Work out the finished part from the listing and answer in its coordinate system (mm). A direction names the side the tool comes from. Round coordinates to 2 decimals unless told otherwise and drop trailing zeros. Loops run counter-clockwise (first coordinate to the right, second up) from the corner with the lowest first, then second, coordinate; pieces in that order, holes last. Notation, with made-up numbers: (23, -3.5) - (45, -3.5) arc R14 cw to (45, 22.5) - close; hole circle Ø10 at (54.5, -16.5). An arc over 180 degrees is marked (long way). Answer as CSV lines item,"result". Start each with the question number.
```python
from build123d import *

# Parameters (mm, degrees)
SKETCH1_R               = 63.5
BOSS_EXTRUDE1_DEPTH     = 25.4
SKETCH2_W               = 190.5
SKETCH2_H               = 190.5
BOSS_EXTRUDE2_DEPTH     = 990.6
BOSS_EXTRUDE3_START     = 25.4
SKETCH3_R               = 63.5
BOSS_EXTRUDE3_DEPTH     = 25.4
SKETCH4_W               = 38.1
SKETCH4_H               = 200.66
BOSS_EXTRUDE4_DEPTH     = 10.16
SKETCH5_R               = 9.525
BOSS_EXTRUDE5_DEPTH     = 4.445
CIRPATTERN3_COUNT       = 4
MIRROR1_COPY_1_SKETCH_W = 38.1
MIRROR1_COPY_1_SKETCH_H = 200.66
MIRROR1_COPY_1_DEPTH    = 10.16
MIRROR1_COPY_2_SKETCH_W = 38.1
MIRROR1_COPY_2_SKETCH_H = 200.66
MIRROR1_COPY_2_DEPTH    = 10.16
MIRROR1_COPY_3_SKETCH_W = 38.1
MIRROR1_COPY_3_SKETCH_H = 200.66
MIRROR1_COPY_3_DEPTH    = 10.16
MIRROR1_COPY_4_SKETCH_R = 9.525
MIRROR1_COPY_4_DEPTH    = 4.445
MIRROR1_COPY_5_SKETCH_R = 9.525
MIRROR1_COPY_5_DEPTH    = 4.445
MIRROR1_COPY_6_SKETCH_R = 9.525
MIRROR1_COPY_6_DEPTH    = 4.445


with BuildPart() as part:
    # Sketch1 → Boss-Extrude1 (new body)
    with BuildSketch(Plane.XY):
        Circle(SKETCH1_R)
    extrude(amount=BOSS_EXTRUDE1_DEPTH)

    # Sketch2 → Boss-Extrude2 (add)
    with BuildSketch(Plane(origin=(0, 0, 0), x_dir=(-1, 0, 0), z_dir=(0, 0, -1))):
        Rectangle(SKETCH2_W, SKETCH2_H)
    extrude(amount=BOSS_EXTRUDE2_DEPTH)

    # Sketch3 → Boss-Extrude3 (add)
    with BuildSketch(Plane(origin=(0, 0, -990.6), x_dir=(-1, 0, 0), z_dir=(0, 0, -1)).offset(BOSS_EXTRUDE3_START)):
        with Locations(Location((0, 0, 0), (0, 0, 180))):
            Circle(SKETCH3_R)
    extrude(amount=-BOSS_EXTRUDE3_DEPTH)

    # Sketch4 → Boss-Extrude4 (add)
    with BuildSketch(Plane(origin=(95.25, 0, 0), x_dir=(0, 0, -1), z_dir=(1, 0, 0))):
        with Locations((31.75, 5.08)):
            Rectangle(SKETCH4_W, SKETCH4_H)
    boss_extrude4 = extrude(amount=BOSS_EXTRUDE4_DEPTH)

    # Sketch5 → Boss-Extrude5 (add)
    with BuildSketch(Plane(origin=(105.41, 0, 0), x_dir=(0, 0, -1), z_dir=(1, 0, 0))):
        with Locations(Location((31.75, 82.55, 0), (0, 0, 180))):
            Circle(SKETCH5_R)
        with Locations(Location((31.75, 41.91, 0), (0, 0, 180))):
            Circle(SKETCH5_R)
        with Locations(Location((31.75, 1.27, 0), (0, 0, 180))):
            Circle(SKETCH5_R)
        with Locations(Location((31.75, -39.37, 0), (0, 0, 180))):
            Circle(SKETCH5_R)
        with Locations(Location((31.75, -80.01, 0), (0, 0, 180))):
            Circle(SKETCH5_R)
    boss_extrude5 = extrude(amount=BOSS_EXTRUDE5_DEPTH)

    # CirPattern3: Boss-Extrude4, Boss-Extrude5 ×4 about axis
    cirpattern3_axis = Axis((0, 0, 0), (0, 0, 1))
    add([boss_extrude4.rotate(cirpattern3_axis, i * 360 / CIRPATTERN3_COUNT) for i in range(1, CIRPATTERN3_COUNT)])
    add([boss_extrude5.rotate(cirpattern3_axis, i * 360 / CIRPATTERN3_COUNT) for i in range(1, CIRPATTERN3_COUNT)])

    # Mirror1: Boss-Extrude4, Boss-Extrude5 across plane
    add(boss_extrude4.mirror(Plane.XY.offset(-495.3)))
    add(boss_extrude5.mirror(Plane.XY.offset(-495.3)))

    # Mirror1 copy 1 sketch → Mirror1 copy 1 (add)
    with BuildSketch(Plane(origin=(0, 95.25, -990.6), x_dir=(0, 0, 1), z_dir=(0, 1, 0))):
        with Locations((31.75, -5.08)):
            Rectangle(MIRROR1_COPY_1_SKETCH_W, MIRROR1_COPY_1_SKETCH_H)
    extrude(amount=MIRROR1_COPY_1_DEPTH)

    # Mirror1 copy 2 sketch → Mirror1 copy 2 (add)
    with BuildSketch(Plane(origin=(-95.25, 0, -990.6), x_dir=(0, 0, 1), z_dir=(-1, 0, 0))):
        with Locations((31.75, -5.08)):
            Rectangle(MIRROR1_COPY_2_SKETCH_W, MIRROR1_COPY_2_SKETCH_H)
    extrude(amount=MIRROR1_COPY_2_DEPTH)

    # Mirror1 copy 3 sketch → Mirror1 copy 3 (add)
    with BuildSketch(Plane(origin=(0, -95.25, -990.6), x_dir=(0, 0, 1), z_dir=(0, -1, 0))):
        with Locations((31.75, -5.08)):
            Rectangle(MIRROR1_COPY_3_SKETCH_W, MIRROR1_COPY_3_SKETCH_H)
    extrude(amount=MIRROR1_COPY_3_DEPTH)

    # Mirror1 copy 4 sketch → Mirror1 copy 4 (add)
    with BuildSketch(Plane(origin=(0, 105.41, -990.6), x_dir=(0, 0, 1), z_dir=(0, 1, 0))):
        with Locations((31.75, -82.55)):
            Circle(MIRROR1_COPY_4_SKETCH_R)
        with Locations((31.75, -41.91)):
            Circle(MIRROR1_COPY_4_SKETCH_R)
        with Locations((31.75, -1.27)):
            Circle(MIRROR1_COPY_4_SKETCH_R)
        with Locations((31.75, 39.37)):
            Circle(MIRROR1_COPY_4_SKETCH_R)
        with Locations((31.75, 80.01)):
            Circle(MIRROR1_COPY_4_SKETCH_R)
    extrude(amount=MIRROR1_COPY_4_DEPTH)

    # Mirror1 copy 5 sketch → Mirror1 copy 5 (add)
    with BuildSketch(Plane(origin=(-105.41, 0, -990.6), x_dir=(0, 0, 1), z_dir=(-1, 0, 0))):
        with Locations((31.75, -82.55)):
            Circle(MIRROR1_COPY_5_SKETCH_R)
        with Locations((31.75, -41.91)):
            Circle(MIRROR1_COPY_5_SKETCH_R)
        with Locations((31.75, -1.27)):
            Circle(MIRROR1_COPY_5_SKETCH_R)
        with Locations((31.75, 39.37)):
            Circle(MIRROR1_COPY_5_SKETCH_R)
        with Locations((31.75, 80.01)):
            Circle(MIRROR1_COPY_5_SKETCH_R)
    extrude(amount=MIRROR1_COPY_5_DEPTH)

    # Mirror1 copy 6 sketch → Mirror1 copy 6 (add)
    with BuildSketch(Plane(origin=(0, -105.41, -990.6), x_dir=(0, 0, 1), z_dir=(0, -1, 0))):
        with Locations((31.75, -82.55)):
            Circle(MIRROR1_COPY_6_SKETCH_R)
        with Locations((31.75, -41.91)):
            Circle(MIRROR1_COPY_6_SKETCH_R)
        with Locations((31.75, -1.27)):
            Circle(MIRROR1_COPY_6_SKETCH_R)
        with Locations((31.75, 39.37)):
            Circle(MIRROR1_COPY_6_SKETCH_R)
        with Locations((31.75, 80.01)):
            Circle(MIRROR1_COPY_6_SKETCH_R)
    extrude(amount=MIRROR1_COPY_6_DEPTH)


solid = part.part
```
Item 1: Flat-ended cylindrical pins translate along their axes: pin 1 Ø12 at (y, z) = (-3, -439) entering from -X; pin 2 Ø1 at (x, y) = (-73.5, -48.5) entering from -Z; pin 3 Ø4 at (y, z) = (22, -3.5) entering from -X. Find the tip coordinate at first contact, or state that the pin passes through.
Item 2: Section A-A, the plane z = -448.5 is taken. Give the vertices of the cut face in (x, y).
Item 3: Determine the mould class of faces 1 (the face through (107.601, 41.491, -949.334)), 2 (the face through (95.25, -1, -489)), 3 (the face through (-109.855, -42, -959)) for opening direction Z: pulls with the +Z half, pulls with the -Z half, needs draft (parallel to the pull), parting line crosses it, or undercut.
Item 4: Find the intervals of material crossed by L1, parallel to Z at x = -100.5, y = 52; L2, parallel to Y at x = 4, z = -172, in increasing order.
Item 5: Which of the six approach directions +Z, -Z, +X, -X, +Y, -Y give full straight-line access (tool end or side, diameter ignored) to faces 4 (the face through (-107.601, -82.131, -968.366)), 5 (the face through (107.601, -39.789, -949.334)), 6 (the face through (-95.25, -1, -489)), 7 (the face through (0.851, -107.601, -41.266))?
Answer:
1,pin 1,"stops at x = -95.25"
1,pin 2,"stops at z = -990.6"
1,pin 3,"stops at x = -95.25"
2,outline,"(-95.25, -95.25) - (95.25, -95.25) - (95.25, 95.25) - (-95.25, 95.25) - close"
3,face 1,"undercut"
3,face 2,"undercut"
3,face 3,"needs draft"
4,L1,"z = -977.9 to -939.8, -50.8 to -12.7"
4,L2,"y = -95.25 to 95.25"
5,face 4,"-X"
5,face 5,"+X"
5,face 6,"-X, +Y, -Y"
5,face 7,"-Y"
